Part model, mm, in its own coordinate system. Coordinates: 2 decimals unless noted, no trailing zeros. Write each loop counter-clockwise with the first axis right and the second up, starting at its lowest first coordinate (ties: lowest second). Pieces come first, ordered by that corner, then holes. Notation, with made-up numbers: (-13.75, 3) -> (13.25, 3) arc R29 cw to (13.25, 28) -> close; hole circle Ø5 at (11, 59.25). An arc over 180 degrees is marked (long way). One line per question, with ' | ' between items. Start each with the question number.
Item 1: Saw through at C-C (z = 12.75). List the corners of the cut face in (x, y), and give its area (3 significant figures).
Item 2: Probe probe 1 along X at (y, z) = (109, 12.25); probe 2 along Y at (x, z) = (-153, 6.75); probe 3 along X at (y, z) = (86, 4.75). List the from-to ranges inside material, lowest first. Write a range as [from, to].
Item 3: Pin check, flat tip, straight feed: pin 1 (1.5 mm diameter, centred on y = 110, z = 3, fed in from -X). Stop position of the tip, or through.
Item 4: Saw through at A-A (z = 2). List the corners of the cut face in (x, y), and give its area (3 significant figures).
Item 5: Saw through at B-B (x = -135.5). List the corners of the cut face in (y, z).
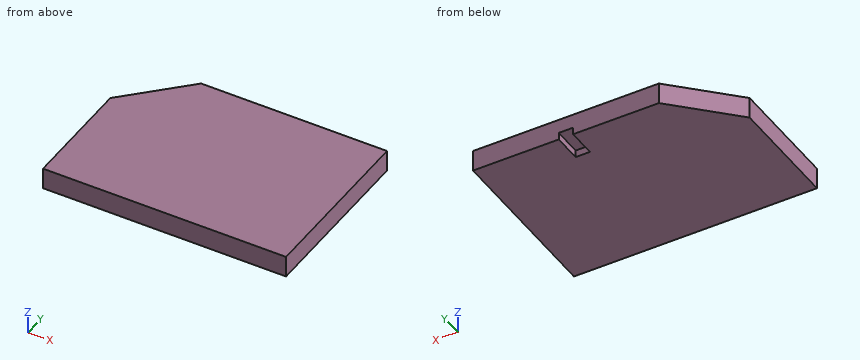
from build123d import *

# Parameters (mm, degrees)
PAD_DEPTH    = 15
SKETCH_W     = 10
SKETCH_H     = 25
POCKET_DEPTH = 5


with BuildPart() as part:
    # CopySketch → Pad (new body)
    with BuildSketch(Plane.XY):
        Polygon((-170, 0), (-170, 80), (-130, 120), (0, 120), (0, 0), align=None)
    extrude(amount=PAD_DEPTH)

    # Sketch (on Face6 of Pad) → Pocket (cut)
    with BuildSketch(Plane(origin=(0, 0, 0), x_dir=(1, 0, 0), z_dir=(0, 0, -1))):
        with Locations((-65, -112.5)):
            Rectangle(SKETCH_W, SKETCH_H)
    extrude(amount=-POCKET_DEPTH, mode=Mode.SUBTRACT)


solid = part.part
From the geometry:
1) outline: (-170, 0) -> (0, 0) -> (0, 120) -> (-130, 120) -> (-170, 80) -> close | area: 19,600 mm2
2) probe 1: [-141, 0] | probe 2: [0, 97] | probe 3: [-164, 0]
3) pin 1: x = -140.75
4) outline: (-170, 0) -> (0, 0) -> (0, 120) -> (-60, 120) -> (-60, 100) -> (-70, 100) -> (-70, 120) -> (-130, 120) -> (-170, 80) -> close | area: 19,400 mm2
5) outline: (0, 0) -> (114.5, 0) -> (114.5, 15) -> (0, 15) -> close
